Can you work these out from the model? Positions are in its coordinate system, mm. A direction names the side the tool comes from. Give positions to 0.01 mm unless a question says otherwise; leave off trailing zeros. Loops run counter-clockwise (first coordinate to the right, second up) from the corner with the lowest first, then second, coordinate; pieces in that order, holes last. Notation, with made-up numbers: (40.25, -40) -> (54.25, -40) arc R20 ccw to (54.25, -2) -> close; hole circle Ø9 at (34.25, 18). An arc over 180 degrees is marked (long way). Return JSON: item names as keys, results as strings. Group by question number.
Q1. I need wall thicknesses on line 1 along Y through (x, z) = (-62.35, -1115); line 2 along Z through (x, y) = (-60.8, 319.75); line 3 along X through (y, z) = (312, -1088). Which ranges of each line are inside material? Lowest first, please. Write a range as [from, to].
Q2. Suppose I cut it at B-B, the plane y = 301. Please give me the cut outline in (x, z), and give its area (3 significant figures).
Q3. Which directions (+Z, -Z, +X, -X, +Y, -Y) give clear straight access to the entire face, cutting with the end or side of a thin tool? Please do faces 1 (the flat face through (-61.6, 278, -1149)), 2 (the cylindrical face through (-64.52, 293.84, -1119.1)).
Q4. Will these pins go through, and if not, where does the flat tip stop? pin 1 (12.5 mm diameter, centred on y = 338.5, z = -1115, fed in from +X); pin 2 (1 mm diameter, centred on x = -69, z = -1102, fed in from +Y); pin 3 (2 mm diameter, centred on x = -60, y = 265.5, fed in from +Z).
Q5. Thinking about a two-plate mould opening in Y: for faces 3 (the flat face through (-61.6, 342, -1118)), 4 (the cylindrical face through (-67.558, 313.69, -1139.397)), which applies, pulls with the +Y half, pulls with the -Y half, needs draft (parallel to the pull), parting line crosses it, or undercut?
Q6. Suppose I cut it at C-C, the plane x = -68.25. Please give me the cut outline in (y, z), and give its area (3 significant figures).
Q7. Suppose I cut it at D-D, the plane z = -1083. Please give me the cut outline in (x, y), and give its area (3 significant figures).
Q8. Suppose I cut it at A-A, the plane z = -1115. Please give me the cut outline in (x, y).
```python
from build123d import *

# Parameters (mm, degrees)
BOSS_EXTRUDE1_OUTLINE_R = 47.5
BOSS_EXTRUDE1_DEPTH     = 6
SKETCH3_R               = 27.5
BOSS_EXTRUDE2_DEPTH     = 6
SKETCH1_3_R             = 4
CUT_EXTRUDE1_DEPTH      = 6
CUT_EXTRUDE2_START      = 3
SKETCH1_4_R             = 7
SKETCH1_4_R_2           = 4
CUT_EXTRUDE2_DEPTH      = 3
CIRPATTERN1_COUNT       = 6
CUT_EXTRUDE3_START      = -58.6
SKETCH4_R               = 8.25
CUT_EXTRUDE3_DEPTH      = 1158.065603692
CUT_EXTRUDE5_DEPTH      = 1216.665603692


# Read off the part's stored shape, not the designer's step: Boss-Extrude1
with BuildPart() as part:
    # Boss-Extrude1 outline → Boss-Extrude1 (new body)
    with BuildSketch(Plane(origin=(-64.6, 0, 0), x_dir=(0, 0, -1), z_dir=(1, 0, 0))):
        with Locations((1115, 301)):
            Circle(BOSS_EXTRUDE1_OUTLINE_R)
    extrude(amount=BOSS_EXTRUDE1_DEPTH)

    # Sketch3 → Boss-Extrude2 (add)
    with BuildSketch(Plane(origin=(-64.6, 0, 0), x_dir=(0, 0, -1), z_dir=(1, 0, 0))):
        with Locations(Location((1115, 301, 0), (0, 0, 90))):
            Circle(SKETCH3_R)
    extrude(amount=-BOSS_EXTRUDE2_DEPTH)

    # Sketch1<3> → Cut-Extrude1 (cut)
    with BuildSketch(Plane(origin=(-64.6, 0, 0), x_dir=(0, 0, -1), z_dir=(1, 0, 0))):
        with Locations(Location((1115, 338.5, 0), (0, 0, 90))):
            Circle(SKETCH1_3_R)
    cut_extrude1 = extrude(amount=CUT_EXTRUDE1_DEPTH, mode=Mode.SUBTRACT)

    # Sketch1<4> → Cut-Extrude2 (cut)
    with BuildSketch(Plane(origin=(-64.6, 0, 0), x_dir=(0, 0, -1), z_dir=(1, 0, 0)).offset(CUT_EXTRUDE2_START)):
        with Locations(Location((1115, 338.5, 0), (0, 0, 90))):
            Circle(SKETCH1_4_R)
        with Locations(Location((1115, 338.5, 0), (0, 0, 90))):
            Circle(SKETCH1_4_R_2, mode=Mode.SUBTRACT)
    cut_extrude2 = extrude(amount=CUT_EXTRUDE2_DEPTH, mode=Mode.SUBTRACT)

    # CirPattern1: Cut-Extrude1, Cut-Extrude2 ×6 about axis
    cirpattern1_axis = Axis((0, 301, -1115), (1, 0, 0))
    add([cut_extrude1.rotate(cirpattern1_axis, i * 360 / CIRPATTERN1_COUNT) for i in range(1, CIRPATTERN1_COUNT)], mode=Mode.SUBTRACT)
    add([cut_extrude2.rotate(cirpattern1_axis, i * 360 / CIRPATTERN1_COUNT) for i in range(1, CIRPATTERN1_COUNT)], mode=Mode.SUBTRACT)

    # Sketch4 → Cut-Extrude3 (cut, through all)
    with BuildSketch(Plane(origin=(0, 0, 0), x_dir=(0, 0, -1), z_dir=(1, 0, 0)).offset(CUT_EXTRUDE3_START)):
        with Locations(Location((1115, 301, 0), (0, 0, 90))):
            Circle(SKETCH4_R)
    extrude(amount=-CUT_EXTRUDE3_DEPTH, mode=Mode.SUBTRACT)

    # Sketch5 → Cut-Extrude5 (cut, through all)
    with BuildSketch(Plane(origin=(0, 0, 0), x_dir=(0, 0, -1), z_dir=(1, 0, 0))):
        with BuildLine():
            Line((1117, 308.745966692), (1117, 310.797958971))
            ThreePointArc((1117, 310.797958971), (1115, 311), (1113, 310.797958971))
            Line((1113, 310.797958971), (1113, 308.745966692))
            ThreePointArc((1113, 308.745966692), (1115, 309), (1117, 308.745966692))
        make_face()
        with BuildLine():
            Line((1122.485281374, 307.631030293), (1120.708203932, 306.605034154))
            ThreePointArc((1120.708203932, 306.605034154), (1121.92820323, 305), (1122.708203932, 303.140932539))
            Line((1122.708203932, 303.140932539), (1124.485281374, 304.166928678))
            ThreePointArc((1124.485281374, 304.166928678), (1123.660254038, 306), (1122.485281374, 307.631030293))
        make_face()
        with BuildLine():
            ThreePointArc((1107.291796067, 303.140932539), (1108.07179677, 305), (1109.291796067, 306.605034154))
            Line((1109.291796067, 306.605034154), (1107.514718626, 307.631030293))
            ThreePointArc((1107.514718626, 307.631030293), (1106.339745962, 306), (1105.514718626, 304.166928678))
            Line((1105.514718626, 304.166928678), (1107.291796067, 303.140932539))
        make_face()
        with BuildLine():
            Line((1124.485281374, 297.833071322), (1122.708203932, 298.859067461))
            ThreePointArc((1122.708203932, 298.859067461), (1121.92820323, 297), (1120.708203932, 295.394965846))
            Line((1120.708203932, 295.394965846), (1122.485281374, 294.368969707))
            ThreePointArc((1122.485281374, 294.368969707), (1123.660254038, 296), (1124.485281374, 297.833071322))
        make_face()
        with BuildLine():
            ThreePointArc((1109.291796067, 295.394965846), (1108.07179677, 297), (1107.291796067, 298.859067461))
            Line((1107.291796067, 298.859067461), (1105.514718626, 297.833071322))
            ThreePointArc((1105.514718626, 297.833071322), (1106.339745962, 296), (1107.514718626, 294.368969707))
            Line((1107.514718626, 294.368969707), (1109.291796067, 295.394965846))
        make_face()
        with BuildLine():
            Line((1117, 291.202041029), (1117, 293.254033308))
            ThreePointArc((1117, 293.254033308), (1115, 293), (1113, 293.254033308))
            Line((1113, 293.254033308), (1113, 291.202041029))
            ThreePointArc((1113, 291.202041029), (1115, 291), (1117, 291.202041029))
        make_face()
    extrude(amount=-CUT_EXTRUDE5_DEPTH, mode=Mode.SUBTRACT)


solid = part.part
```
Ans:
{
 "1": {"line 1": "y = [253.5, 259.5], [267.5, 291], [311, 334.5], [342.5, 348.5]", "line 2": "z = [-1158.64, -1154.48], [-1140.48, -1089.52], [-1075.52, -1071.36]", "line 3": "x = [-64.6, -58.6]"},
 "2": {"outline": "(-70.6, -1142.5) -> (-64.6, -1142.5) -> (-64.6, -1162.5) -> (-58.6, -1162.5) -> (-58.6, -1123.25) -> (-70.6, -1123.25) -> close; (-70.6, -1106.75) -> (-58.6, -1106.75) -> (-58.6, -1067.5) -> (-64.6, -1067.5) -> (-64.6, -1087.5) -> (-70.6, -1087.5) -> close", "area": "702 mm^2"},
 "3": {"face 1": "+X", "face 2": "+X, -X"},
 "4": {"pin 1": "stops at x = -61.6", "pin 2": "stops at y = 325.49", "pin 3": "stops at z = -1082.35"},
 "5": {"face 3": "undercut", "face 4": "parting line crosses it"},
 "6": {"outline": "circle Ø55 at (301, -1115); hole (291.2, -1117) -> (293, -1117) arc R8.25 ccw to (295.27, -1120.93) -> (294.37, -1122.49) arc R10 ccw to (297.83, -1124.49) -> (298.73, -1122.93) arc R8.25 ccw to (303.27, -1122.93) -> (304.17, -1124.49) arc R10 ccw to (307.63, -1122.49) -> (306.73, -1120.93) arc R8.25 ccw to (309, -1117) -> (310.8, -1117) arc R10 ccw to (310.8, -1113) -> (309, -1113) arc R8.25 ccw to (306.73, -1109.07) -> (307.63, -1107.51) arc R10 ccw to (304.17, -1105.51) -> (303.27, -1107.07) arc R8.25 ccw to (298.73, -1107.07) -> (297.83, -1105.51) arc R10 ccw to (294.37, -1107.51) -> (295.27, -1109.07) arc R8.25 ccw to (293, -1113) -> (291.2, -1113) arc R10 ccw to start", "area": "2,120 mm^2"},
 "7": {"outline": "(-64.6, 265.9) -> (-58.6, 265.9) -> (-58.6, 275.27) -> (-61.6, 275.27) -> (-61.6, 278.28) -> (-64.6, 278.28) -> close; (-64.6, 286.22) -> (-61.6, 286.22) -> (-61.6, 289.23) -> (-58.6, 289.23) -> (-58.6, 312.77) -> (-61.6, 312.77) -> (-61.6, 315.78) -> (-64.6, 315.78) -> close; (-64.6, 323.72) -> (-61.6, 323.72) -> (-61.6, 326.73) -> (-58.6, 326.73) -> (-58.6, 336.1) -> (-64.6, 336.1) -> close", "area": "290 mm^2"},
 "8": {"outline": "(-70.6, 273.5) -> (-64.6, 273.5) -> (-64.6, 267.5) -> (-61.6, 267.5) -> (-61.6, 270.5) -> (-58.6, 270.5) -> (-58.6, 291) -> (-70.6, 291) -> close; (-70.6, 311) -> (-58.6, 311) -> (-58.6, 331.5) -> (-61.6, 331.5) -> (-61.6, 334.5) -> (-64.6, 334.5) -> (-64.6, 328.5) -> (-70.6, 328.5) -> close; (-64.6, 253.5) -> (-58.6, 253.5) -> (-58.6, 256.5) -> (-61.6, 256.5) -> (-61.6, 259.5) -> (-64.6, 259.5) -> close; (-64.6, 342.5) -> (-61.6, 342.5) -> (-61.6, 345.5) -> (-58.6, 345.5) -> (-58.6, 348.5) -> (-64.6, 348.5) -> close"}
}
